Build history of the part. All positions in model axes, mm. A direction names the side the tool comes from. Round coordinates to 2 decimals unless told otherwise and drop trailing zeros. Write each loop counter-clockwise with the first axis right and the second up, starting at its lowest first coordinate (ties: lowest second). Pieces come first, ordered by that corner, then holes. Notation, with made-up numbers: (-14, -12.75) -> (23, -12.75) arc R30 ccw to (23, 12.25) -> close; hole circle Ø4 at (79, -35.5). An arc over 180 degrees is marked (long way). Answer as CSV lines item,"result".
Autodesk Inventor part; units mm, degrees
ref_plane "YZ Plane" through (0, 0, 0) normal (1, 0, 0) x (0, 1, 0)
ref_plane "XZ Plane" through (0, 0, 0) normal (0, 1, 0) x (-1, 0, 0)
ref_plane "XY Plane" through (0, 0, 0) normal (0, 0, 1) x (1, 0, 0)
ref_plane "Work Plane1" through (0, 0, 0) normal (0, 0, 1) x (1, 0, 0)
sketch "Sketch1" plane through (0, 0, 0) normal (0, 0, 1) x (1, 0, 0)
  circle A0 centre (11.8906, 0.2887) radius 14 construction
  line L0 (-4.1094, 7.6362) -> (-12.7094, 0.2473) construction
  line L1 (-5.7094, 0.2473) -> (-12.7094, 0.2473) construction
  line L2 (-5.7094, -6.0861) -> (-5.7094, 0.2473) construction
  line L3 (-6.0301, -6.0861) -> (-5.7094, -6.0861) construction
  line L4 (-6.0301, -6.0861) -> (-4.1094, -7.5697) construction
  line L5 (-4.1094, -7.5697) -> (-4.1094, -15.7113) construction
  line L6 (-4.1094, -15.7113) -> (27.8906, -15.7113) construction
  line L7 (27.8906, -15.7113) -> (27.8906, -7.5697) construction
  line L8 (29.8113, -6.0861) -> (27.8906, -7.5697) construction
  line L9 (29.4906, -6.0861) -> (29.8113, -6.0861) construction
  line L10 (29.4906, 0.2473) -> (29.4906, -6.0861) construction
  line L11 (36.4906, 0.2473) -> (29.4906, 0.2473) construction
  line L12 (27.8906, 7.6362) -> (36.4906, 0.2473) construction
  line L13 (27.8906, 7.6362) -> (27.8906, 16.2887) construction
  line L14 (27.8906, 16.2887) -> (-4.1094, 16.2887) construction
  line L15 (-4.1094, 16.2887) -> (-4.1094, 7.6362) construction
  circle A1 centre (11.8906, 0.2887) radius 13.9
  circle A2 centre (11.8906, 0.2887) radius 12.5
  point P0 (0, 0)
  dimension "d0" = 27.8
  dimension "d1" = 25
extrude "Extrusion1" add sketch "Sketch1" against normal blind 3 draft -2
sketch "Sketch2" plane through (11.8906, 0.2887, 0) normal (0, 0, 1) x (1, 0, 0)
  circle A0 centre (0, 0) radius 13.9
  circle A1 centre (0, 0) radius 12.5
  line L0 (17, -14) -> (-17, -14)
  line L1 (-17, -14) -> (-17, 14)
  line L2 (-17, 14) -> (17, 14)
  line L3 (17, 14) -> (17, -14)
  line L4 (17, -14) -> (-17, 14) construction
  line L5 (-17, -14) -> (17, 14) construction
  circle A2 centre (0, 0) radius 10.05 construction
  line L6 (-7.4329, 10.05) -> (7.4329, 10.05)
  line L7 (-12.42, 1.4121) -> (-4.9871, -11.4621)
  line L8 (4.9871, -11.4621) -> (12.42, 1.4121)
  point P0 (-11.8906, -0.2887)
  dimension "d4" = 34
  dimension "d5" = 28
  dimension "d8" = 20.1
  dimension "d9" = 60
  dimension "d10" = 60
  dimension "d11" = 0
extrude "Extrusion2" add sketch "Sketch2" along normal blind 2 contours A0 | A1 L8 | L6 A1 | A1 L7 | L0 L1 L2 L3
properties part number "20_Cube_Insert_Z-Focus_objectivemount"
1. Mould opens along X. For faces 4 (the flat face through (3.135, -4.646, 0.986)), 5 (the flat face through (-5.109, 0, 1)), 6 (the flat face through (19, -12, 0)) say: +X half, -X half, draft (parallel to the pull), parting line (faces both ways), or undercut.
Results found:
face 4,"undercut"
face 5,"-X half"
face 6,"draft"
2. Which spindle directions (+Z, -Z, +X, -X, +Y, -Y) get a long thin tool onto all of the face, cutting with end or side? Do faces 1 (the flat face through (18, -11, -3)), 2 (the flat face through (21, -5, 0)), 3 (the cylindrical face through (11.96, -12.21, 0.99)). Say none if no direction does.
Results found:
face 1,"-Z, +X, -X, +Y, -Y"
face 2,"-Z"
face 3,"+Z, -Z"
3. Probe line 1 along Z through (x, y) = (-2, 6.5); line 2 along X through (y, z) = (9.5, 0.75); line 3 along Y through (x, z) = (8, 0.1). List the from-to ranges inside material, lowest first.
Results found:
line 1,"z = 0 to 2"
line 2,"x = -5.11 to 3.44, 20.34 to 28.89"
line 3,"y = -13.71 to -11.59, 10.34 to 14.29"
4. Cut at B-B, the plane z = -1.1. Write the cut outline in (x, y), then the cut area to 3 significant figures.
Results found:
outline,"circle Ø27.72 at (11.89, 0.29); hole circle Ø25.08 at (11.89, 0.29)"
area,"110 mm2"
5. Cut at A-A, the plane z = 1.4. Write the cut outline in (x, y), then the cut area to 3 significant figures.
Results found:
outline,"(-5.11, -13.71) -> (28.89, -13.71) -> (28.89, 14.29) -> (-5.11, 14.29) -> close; hole (-0.53, 1.7) -> (6.9, -11.17) arc R12.5 ccw to (16.88, -11.17) -> (24.31, 1.7) arc R12.5 ccw to (19.32, 10.34) -> (4.46, 10.34) arc R12.5 ccw to start"
area,"536 mm2"
6. Drop flat-ended pins along their axis: pin 1 Ø2 at (y, z) = (1.5, -2) entering from -X; pin 2 Ø0.7 at (x, y) = (8.5, 11.5) entering from -Z; pin 3 Ø8 at (x, y) = (10, -1) entering from +Z. Give the stop position or say it passes through.
Results found:
pin 1,"stops at x = -1.96"
pin 2,"stops at z = 0"
pin 3,"passes through"
